Source: CAD feature listing. Evaluate the final solid. Frame: model axes, mm. A direction names the side the tool comes from. Round coordinates to 2 decimals unless told otherwise and drop trailing zeros. Loops run counter-clockwise (first coordinate to the right, second up) from the corner with the lowest first, then second, coordinate; pieces in that order, holes last.
Item 1: Section query D-D on x = 13. Return loops of the section in (y, z), then the cut area to 3 significant figures.
Item 2: Ray query, L1, parallel to Y at x = 60, z = 1.6; L2, parallel to X at y = -1, z = 1.9; L3, parallel to X at y = 1.5, z = 0.75. Return the intervals inside material, ascending.
Item 3: Section query A-A on x = 0. Return loops of the section in (y, z).
Item 4: Access query for faces 4 (the flat face through (30, 3, 2)), 5 (the flat face through (30, 0.75, 1)). Directions: +Z, -Z, +X, -X, +Y, -Y. A direction counts if a zero-diameter tool reaches every point of the face in a straight line with its end or side. Return the directions, or none.
Item 5: Section query C-C on y = 3.25. Return loops of the section in (x, z).
Item 6: Section query B-B on z = 0.75. Return loops of the section in (x, y), then the cut area to 3 significant figures.
Item 7: Pull-direction query (Y, two-part tool) for faces 1 (the cylindrical face through (4.621, 5.075, 0.986)), 2 (the cylindrical face through (-3.816, -2.385, 0.986)), 3 (the cylindrical face through (61.617, -0.67, 0.986)); classes: released by +Y, released by -Y, zero draft, split by the parting line, or undercut.
```python
from build123d import *

# Parameters (mm, degrees)
SKETCH1_R           = 1.75
BOSS_EXTRUDE1_DEPTH = 2


with BuildPart() as part:
    # Sketch1 → Boss-Extrude1 (new body)
    with BuildSketch(Plane.XY):
        with BuildLine():
            Line((2.717606537, 4.167087077), (3.433012702, 4.580127019))
            ThreePointArc((3.433012702, 4.580127019), (4.638917476, 5.079629131), (5.933012702, 5.25))
            Line((5.933012702, 5.25), (54.066987298, 5.25))
            ThreePointArc((54.066987298, 5.25), (55.361082524, 5.079629131), (56.566987298, 4.580127019))
            Line((56.566987298, 4.580127019), (57.282393463, 4.167087077))
            ThreePointArc((57.282393463, 4.167087077), (57.728126896, 4.034585997), (58.185594651, 4.118001121))
            ThreePointArc((58.185594651, 4.118001121), (63.897114317, -2.25), (55.526503742, -0.487679436))
            ThreePointArc((55.526503742, -0.487679436), (55.370009481, -0.049793176), (55.032393463, 0.26997276))
            Line((55.032393463, 0.26997276), (54.665063509, 0.482050808))
            ThreePointArc((54.665063509, 0.482050808), (54.1827016, 0.681851653), (53.665063509, 0.75))
            Line((53.665063509, 0.75), (6.350969201, 0.75))
            ThreePointArc((6.350969201, 0.75), (5.817844702, 0.679812828), (5.321051756, 0.474034452))
            Line((5.321051756, 0.474034452), (4.967606537, 0.26997276))
            ThreePointArc((4.967606537, 0.26997276), (4.629990519, -0.049793176), (4.473496258, -0.487679436))
            ThreePointArc((4.473496258, -0.487679436), (-3.897114317, -2.25), (1.814405349, 4.118001121))
            ThreePointArc((1.814405349, 4.118001121), (2.271873104, 4.034585997), (2.717606537, 4.167087077))
        make_face()
        Circle(SKETCH1_R, mode=Mode.SUBTRACT)
        with Locations((60, 0)):
            Circle(SKETCH1_R, mode=Mode.SUBTRACT)
    extrude(amount=BOSS_EXTRUDE1_DEPTH)


solid = part.part
```
Data:
1. outline: (0.75, 0) - (5.25, 0) - (5.25, 2) - (0.75, 2) - close
1. area: 9.00 mm2
2. L1: y = -4.5 to -1.75, 1.75 to 4.5
2. L2: x = -4.39 to -1.44, 1.44 to 4.39, 55.61 to 58.56, 61.44 to 64.39
2. L3: x = -4.24 to -0.9, 0.9 to 59.1, 60.9 to 64.24
3. outline: (-4.5, 0) - (-1.75, 0) - (-1.75, 2) - (-4.5, 2) - close; (1.75, 0) - (4.5, 0) - (4.5, 2) - (1.75, 2) - close
4. face 4: +Z, +X, -X, +Y, -Y
4. face 5: +Z, -Z, -Y
5. outline: (-3.11, 0) - (63.11, 0) - (63.11, 2) - (-3.11, 2) - close
6. outline: (1.81, 4.12) arc R4.5 ccw (long way) to (4.47, -0.49) arc R1 cw to (4.97, 0.27) - (5.32, 0.47) arc R2.06 cw to (6.35, 0.75) - (53.67, 0.75) arc R2 cw to (54.67, 0.48) - (55.03, 0.27) arc R1 cw to (55.53, -0.49) arc R4.5 ccw (long way) to (58.19, 4.12) arc R1 cw to (57.28, 4.17) - (56.57, 4.58) arc R5 ccw to (54.07, 5.25) - (5.93, 5.25) arc R5 ccw to (3.43, 4.58) - (2.72, 4.17) arc R1 cw to start; hole circle Ø3.5 at (0, 0); hole circle Ø3.5 at (60, 0)
6. area: 346 mm2
7. face 1: released by +Y
7. face 2: split by the parting line
7. face 3: undercut
